```python
from build123d import *

# Parameters (mm, degrees)
SKETCH1_R           = 10.85
BOSS_EXTRUDE1_DEPTH = 6
SCALE1_SCALE        = 0.4


with BuildPart() as part:
    # Sketch1 → Boss-Extrude1 (new body)
    with BuildSketch(Plane.XY):
        with Locations((3, 0)):
            Circle(SKETCH1_R)
        Polygon((0, 5.773502692), (-5, 2.886751346), (-5, -2.886751346), (0, -5.773502692), (5, -2.886751346), (5, 2.886751346), align=None, mode=Mode.SUBTRACT)
    extrude(amount=-BOSS_EXTRUDE1_DEPTH)


with BuildPart() as part_1:
    # Scale1: scaled about (3.917290958, 0, -3)
    add(part.part.scale(SCALE1_SCALE).moved(Location((2.350374575, 0, -1.8))))


solid = part_1.part
```
CAD build for the part. Positions are in the model's coordinates, mm. A direction names the side the tool comes from. Round coordinates to 2 decimals unless told otherwise and drop trailing zeros. Loops run counter-clockwise (first coordinate to the right, second up) from the corner with the lowest first, then second, coordinate; pieces in that order, holes last. Notation, with made-up numbers: M 30.5,12 L 81.5,12 A21 cw 81.5,41 Z; hole C -34.75,61.25 d1. An arc over 180 degrees is marked long. Use a Markdown table: item, result. Add a question column.
(1) Cut at A-A (y = 0). Give the cut face in (x, z), and give its area (3 significant figures).
(2) Cut at D-D (x = 6.75). Give the cut face in (y, z), and give its area (3 significant figures).
(3) Which spindle directions (+Z, -Z, +X, -X, +Y, -Y) get a long thin tool onto all of the face, cutting with end or side? Do faces 1 (the face through (5, 0, -4.2)), 2 (the face through (1.336, -1.724, -2.983)). Say none if no direction does.
(4) Cut at B-B (z = -2.9). Give the cut face in (x, y), and give its area (3 significant figures).
(5) Drill centre lines: line 1 (X direction, y = 1.5, z = -1.9); line 2 (X direction, y = 0.5, z = -2.75); line 3 (Y direction, x = 1.25, z = -2.5). Where is each one in solid material? Low to high.
(6) Pull direction Y, two halves, no side cores. Call faces 3 (the face through (7.69, 1.3, -2.98)), 4 (the face through (5, 0, -1.8)), 5 (the face through (0.35, 0, -3)): +Y half, -Y half, draft (parallel to the pull), parting line (faces both ways), or undercut.
(7) Cut at C-C (x = 3.5). Give the cut face in (y, z).
Geometry says:
| question | item | result |
|---|---|---|
| 1 | outline | M -0.79,-4.2 L 0.35,-4.2 L 0.35,-1.8 L -0.79,-1.8 Z; M 4.35,-4.2 L 7.89,-4.2 L 7.89,-1.8 L 4.35,-1.8 Z |
| 1 | area | 11.2 mm² |
| 2 | outline | M -2.93,-4.2 L 2.93,-4.2 L 2.93,-1.8 L -2.93,-1.8 Z |
| 2 | area | 14.1 mm² |
| 3 | face 1 | -Z, +X, -X, +Y, -Y |
| 3 | face 2 | +Z, -Z |
| 4 | outline | C 3.55,0 d8.68; hole M 0.35,-1.15 L 2.35,-2.31 L 4.35,-1.15 L 4.35,1.15 L 2.35,2.31 L 0.35,1.15 Z |
| 4 | area | 45.3 mm² |
| 5 | line 1 | x = -0.52 to 0.95, 3.75 to 7.62 |
| 5 | line 2 | x = -0.76 to 0.35, 4.35 to 7.86 |
| 5 | line 3 | y = -3.68 to -1.67, 1.67 to 3.68 |
| 6 | face 3 | parting line |
| 6 | face 4 | draft |
| 6 | face 5 | undercut |
| 7 | outline | M -4.34,-4.2 L -1.65,-4.2 L -1.65,-1.8 L -4.34,-1.8 Z; M 1.65,-4.2 L 4.34,-4.2 L 4.34,-1.8 L 1.65,-1.8 Z |
